Read the model definition and answer for the solid it produces. Units are mm, in the model's axes. A direction names the side the tool comes from. Give positions to 0.01 mm unless a question says otherwise; leave off trailing zeros. Write each loop counter-clockwise with the first axis right and the second up, starting at its lowest first coordinate (ties: lowest second). Pieces come first, ordered by that corner, then holes. Notation, with made-up numbers: M 1,-27.75 L 27,-27.75 A32 cw 27,4.25 Z; hole C 65.25,-11.5 d3. An arc over 180 degrees is marked long. Use a Markdown table: item, result. Add a question column.
Item 1: For faces 1 (the cylindrical face through (9.71, 2.96, 7.05)), 2 (the cylindrical face through (-3.71, 2.96, -11.41)), 3 (the flat face through (-9.325, 2.958, 5.852)), determine the directions among +Z, -Z, +X, -X, +Y, -Y from which every point of the face is accessible in a straight line to the end or side of a thin tool.
Item 2: The mould has two halves that part along Y. Classify faces 4 (the flat face through (4.2, 0, -9.4)), 5 (the cylindrical face through (12.932, -0.986, 5.362)): pulls with the +Y half, pulls with the -Y half, needs draft (parallel to the pull), parting line crosses it, or undercut.
Item 3: A cutting plane is placed at B-B on z = 0. Determine the outline of the cut face in (x, y).
Item 4: Consider probe 1 along Y at (x, z) = (-11.5, -4.5); probe 2 along Z at (x, y) = (0, 7.5); probe 3 along X at (y, z) = (3.4, 0). Determine where each line is inside the solid, lowest interval first. Write a range as [from, to].
Item 5: Given P1, Ø4, axis at x = 0, z = 0, coming from the -Y side; P2, Ø1, axis at y = 5, z = -0.5, coming from the +X side; P3, Ø8, axis at x = 0, z = 0, coming from the +Y side; P4, Ø1.5, axis at y = 2.5, z = 10.5, coming from the +X side, each flat-ended and moving along its own axis, determine where each tip first touches the part or whether it passes through.
Item 6: A cutting plane is placed at C-C on y = -0.5. Determine the outline of the cut face in (x, z).
Item 7: A cutting plane is placed at A-A on x = 0. Determine the outline of the cut face in (y, z).
from build123d import *

# Parameters (mm, degrees)
SKETCH1_R           = 2.5
BOSS_EXTRUDE1_DEPTH = 6
SKETCH2_W           = 11.45
SKETCH2_H           = 2
SKETCH3_R           = 5
CUT_EXTRUDE1_DEPTH  = 1


with BuildPart() as part:
    # Sketch1 → Boss-Extrude1 (new body)
    with BuildSketch(Plane(origin=(0, 0, 0), x_dir=(1, 0, 0), z_dir=(0, 1, 0))):
        with BuildLine():
            Line((0.5, 11.989578808), (1, 9.949874371))
            ThreePointArc((1, 9.949874371), (1.56434465, 9.876883406), (2.123623756, 9.771909851))
            Line((2.123623756, 9.771909851), (3.229455349, 11.55727555))
            ThreePointArc((3.229455349, 11.55727555), (3.708203932, 11.412678196), (4.180511865, 11.248258556))
            Line((4.180511865, 11.248258556), (4.025736789, 9.153875863))
            ThreePointArc((4.025736789, 9.153875863), (4.539904997, 8.910065242), (5.039372423, 8.63740271))
            Line((5.039372423, 8.63740271), (6.642789108, 9.993665637))
            ThreePointArc((6.642789108, 9.993665637), (7.053423028, 9.708203932), (7.451806102, 9.405880385))
            Line((7.451806102, 9.405880385), (6.657406412, 7.461832206))
            ThreePointArc((6.657406412, 7.461832206), (7.071067812, 7.071067812), (7.461832206, 6.657406412))
            Line((7.461832206, 6.657406412), (9.405880385, 7.451806102))
            ThreePointArc((9.405880385, 7.451806102), (9.708203932, 7.053423028), (9.993665637, 6.642789108))
            Line((9.993665637, 6.642789108), (8.63740271, 5.039372423))
            ThreePointArc((8.63740271, 5.039372423), (8.910065242, 4.539904997), (9.153875863, 4.025736789))
            Line((9.153875863, 4.025736789), (11.248258556, 4.180511865))
            ThreePointArc((11.248258556, 4.180511865), (11.412678196, 3.708203932), (11.55727555, 3.229455349))
            Line((11.55727555, 3.229455349), (9.771909851, 2.123623756))
            ThreePointArc((9.771909851, 2.123623756), (9.876883406, 1.56434465), (9.949874371, 1))
            Line((9.949874371, 1), (11.989578808, 0.5))
            ThreePointArc((11.989578808, 0.5), (12, 0), (11.989578808, -0.5))
            Line((11.989578808, -0.5), (9.949874371, -1))
            ThreePointArc((9.949874371, -1), (9.876883406, -1.56434465), (9.771909851, -2.123623756))
            Line((9.771909851, -2.123623756), (11.55727555, -3.229455349))
            ThreePointArc((11.55727555, -3.229455349), (11.412678196, -3.708203932), (11.248258556, -4.180511865))
            Line((11.248258556, -4.180511865), (9.153875863, -4.025736789))
            ThreePointArc((9.153875863, -4.025736789), (8.910065242, -4.539904997), (8.63740271, -5.039372423))
            Line((8.63740271, -5.039372423), (9.993665637, -6.642789108))
            ThreePointArc((9.993665637, -6.642789108), (9.708203932, -7.053423028), (9.405880385, -7.451806102))
            Line((9.405880385, -7.451806102), (7.461832206, -6.657406412))
            ThreePointArc((7.461832206, -6.657406412), (7.071067812, -7.071067812), (6.657406412, -7.461832206))
            Line((6.657406412, -7.461832206), (7.451806102, -9.405880385))
            ThreePointArc((7.451806102, -9.405880385), (7.053423028, -9.708203932), (6.642789108, -9.993665637))
            Line((6.642789108, -9.993665637), (5.039372423, -8.63740271))
            ThreePointArc((5.039372423, -8.63740271), (4.539904997, -8.910065242), (4.025736789, -9.153875863))
            Line((4.025736789, -9.153875863), (4.180511865, -11.248258556))
            ThreePointArc((4.180511865, -11.248258556), (3.708203932, -11.412678196), (3.229455349, -11.55727555))
            Line((3.229455349, -11.55727555), (2.123623756, -9.771909851))
            ThreePointArc((2.123623756, -9.771909851), (1.56434465, -9.876883406), (1, -9.949874371))
            Line((1, -9.949874371), (0.5, -11.989578808))
            ThreePointArc((0.5, -11.989578808), (0, -12), (-0.5, -11.989578808))
            Line((-0.5, -11.989578808), (-1, -9.949874371))
            ThreePointArc((-1, -9.949874371), (-1.56434465, -9.876883406), (-2.123623756, -9.771909851))
            Line((-2.123623756, -9.771909851), (-3.229455349, -11.55727555))
            ThreePointArc((-3.229455349, -11.55727555), (-3.708203932, -11.412678196), (-4.180511865, -11.248258556))
            Line((-4.180511865, -11.248258556), (-4.025736789, -9.153875863))
            ThreePointArc((-4.025736789, -9.153875863), (-4.539904997, -8.910065242), (-5.039372423, -8.63740271))
            Line((-5.039372423, -8.63740271), (-6.642789108, -9.993665637))
            ThreePointArc((-6.642789108, -9.993665637), (-7.053423028, -9.708203932), (-7.451806102, -9.405880385))
            Line((-7.451806102, -9.405880385), (-6.657406412, -7.461832206))
            ThreePointArc((-6.657406412, -7.461832206), (-7.071067812, -7.071067812), (-7.461832206, -6.657406412))
            Line((-7.461832206, -6.657406412), (-9.405880385, -7.451806102))
            ThreePointArc((-9.405880385, -7.451806102), (-9.708203932, -7.053423028), (-9.993665637, -6.642789108))
            Line((-9.993665637, -6.642789108), (-8.63740271, -5.039372423))
            ThreePointArc((-8.63740271, -5.039372423), (-8.910065242, -4.539904997), (-9.153875863, -4.025736789))
            Line((-9.153875863, -4.025736789), (-11.248258556, -4.180511865))
            ThreePointArc((-11.248258556, -4.180511865), (-11.412678196, -3.708203932), (-11.55727555, -3.229455349))
            Line((-11.55727555, -3.229455349), (-9.771909851, -2.123623756))
            ThreePointArc((-9.771909851, -2.123623756), (-9.876883406, -1.56434465), (-9.949874371, -1))
            Line((-9.949874371, -1), (-11.989578808, -0.5))
            ThreePointArc((-11.989578808, -0.5), (-12, 0), (-11.989578808, 0.5))
            Line((-11.989578808, 0.5), (-9.949874371, 1))
            ThreePointArc((-9.949874371, 1), (-9.876883406, 1.56434465), (-9.771909851, 2.123623756))
            Line((-9.771909851, 2.123623756), (-11.55727555, 3.229455349))
            ThreePointArc((-11.55727555, 3.229455349), (-11.412678196, 3.708203932), (-11.248258556, 4.180511865))
            Line((-11.248258556, 4.180511865), (-9.153875863, 4.025736789))
            ThreePointArc((-9.153875863, 4.025736789), (-8.910065242, 4.539904997), (-8.63740271, 5.039372423))
            Line((-8.63740271, 5.039372423), (-9.993665637, 6.642789108))
            ThreePointArc((-9.993665637, 6.642789108), (-9.708203932, 7.053423028), (-9.405880385, 7.451806102))
            Line((-9.405880385, 7.451806102), (-7.461832206, 6.657406412))
            ThreePointArc((-7.461832206, 6.657406412), (-7.071067812, 7.071067812), (-6.657406412, 7.461832206))
            Line((-6.657406412, 7.461832206), (-7.451806102, 9.405880385))
            ThreePointArc((-7.451806102, 9.405880385), (-7.053423028, 9.708203932), (-6.642789108, 9.993665637))
            Line((-6.642789108, 9.993665637), (-5.039372423, 8.63740271))
            ThreePointArc((-5.039372423, 8.63740271), (-4.539904997, 8.910065242), (-4.025736789, 9.153875863))
            Line((-4.025736789, 9.153875863), (-4.180511865, 11.248258556))
            ThreePointArc((-4.180511865, 11.248258556), (-3.708203932, 11.412678196), (-3.229455349, 11.55727555))
            Line((-3.229455349, 11.55727555), (-2.123623756, 9.771909851))
            ThreePointArc((-2.123623756, 9.771909851), (-1.56434465, 9.876883406), (-1, 9.949874371))
            Line((-1, 9.949874371), (-0.5, 11.989578808))
            ThreePointArc((-0.5, 11.989578808), (0, 12), (0.5, 11.989578808))
        make_face()
        with Locations(Location((0, 0, 0), (0, 0, 270))):
            Circle(SKETCH1_R, mode=Mode.SUBTRACT)
    extrude(amount=BOSS_EXTRUDE1_DEPTH)

    # Sketch2 → Revolve1 (revolve)
    with BuildSketch(Plane.XY):
        with Locations((8.275, -1)):
            Rectangle(SKETCH2_W, SKETCH2_H)
        with Locations((8.275, 7)):
            Rectangle(SKETCH2_W, SKETCH2_H)
    revolve(axis=Axis((0, -1000, 0), (0, 1, 0)))

    # Sketch3 → Cut-Extrude1 (cut)
    with BuildSketch(Plane(origin=(0, 8, 0), x_dir=(1, 0, 0), z_dir=(0, 1, 0))):
        with Locations(Location((0, 0, 0), (0, 0, 180))):
            Circle(SKETCH3_R)
    extrude(amount=-CUT_EXTRUDE1_DEPTH, mode=Mode.SUBTRACT)


solid = part.part
Filled in:
| question | item | result |
|---|---|---|
| 1 | face 1 | +Z, +X |
| 1 | face 2 | -Z, -X |
| 1 | face 3 | -X |
| 2 | face 4 | undercut |
| 2 | face 5 | needs draft |
| 3 | outline | M -14,-2 L -2.55,-2 L -2.55,0 L -2.5,0 L -2.5,6 L -2.55,6 L -2.55,7 L -5,7 L -5,8 L -14,8 L -14,6 L -12,6 L -12,0 L -14,0 Z; M 2.5,0 L 2.55,0 L 2.55,-2 L 14,-2 L 14,0 L 12,0 L 12,6 L 14,6 L 14,8 L 5,8 L 5,7 L 2.55,7 L 2.55,6 L 2.5,6 Z |
| 4 | probe 1 | [-2, 0], [6, 8] |
| 4 | probe 2 | [-14, -5], [5, 14] |
| 4 | probe 3 | [-12, -2.5], [2.5, 12] |
| 5 | P1 | through |
| 5 | P2 | x = 12 |
| 5 | P3 | y = 7 |
| 5 | P4 | x = 7 |
| 6 | outline | C 0,0 d28; hole C 0,0 d5.1 |
| 7 | outline | M -2,-14 L 0,-14 L 0,-12 L 6,-12 L 6,-14 L 8,-14 L 8,-5 L 7,-5 L 7,-2.55 L 6,-2.55 L 6,-2.5 L 0,-2.5 L 0,-2.55 L -2,-2.55 Z; M -2,2.55 L 0,2.55 L 0,2.5 L 6,2.5 L 6,2.55 L 7,2.55 L 7,5 L 8,5 L 8,14 L 6,14 L 6,12 L 0,12 L 0,14 L -2,14 Z |
